Part model, mm, in its own coordinate system. Face numbers are marked on the shaded views. A direction names the side the tool comes from. Round coordinates to 2 decimals unless told otherwise and drop trailing zeros. Write each loop counter-clockwise with the first axis right and the second up, starting at its lowest first coordinate (ties: lowest second). Pieces come first, ordered by that corner, then holes. Notation, with made-up numbers: M 78.25,-7 L 132.25,-7 A31 ccw 132.25,28 Z; hole C -9.75,27.5 d6. An arc over 180 degrees is marked long. Use one line per item in the form item = value. Start each with the question number.
Item 1: Which spindle directions (+Z, -Z, +X, -X, +Y, -Y) get a long thin tool onto all of the face, cutting with end or side? Do the marked faces 5, 6, 7 and 8. Say none if no direction does.
Item 2: Cut at C-C, the plane z = 10.75. Give the cut face in (x, y).
Item 3: Mould opens along Y. For the marked faces 1, 2, 3 and 4 say: +Y half, -Y half, draft (parallel to the pull), parting line (faces both ways), or undercut.
Item 4: Cut at D-D, the plane y = 17. Give the cut face in (x, z).
Item 5: Cut at A-A, the plane z = 4.75. Give the cut face in (x, y).
Item 6: Probe L1, parallel to Y at x = -3, z = 2.5; L2, parallel to X at y = 24.5, z = 3; L3, parallel to Y at x = -18, z = 0.75. List the from-to ranges inside material, lowest first.
Item 7: Flat gauge pins, fed straight in: pin 1 Ø4 at (y, z) = (19, 7.5) entering from +X; pin 2 Ø1.5 at (x, y) = (-5, 18.5) entering from -Z; pin 3 Ø3 at (x, y) = (-20.5, -7) entering from +Z; pin 4 Ø1.2 at (y, z) = (-25.5, 1) entering from +X. Where does each tip first touch, or does it go through?
Item 8: Cut at B-B, the plane x = -4.5. Give the cut face in (y, z), then the cut area to 4 significant figures.
from build123d import *

# Parameters (mm, degrees)
F0_R     = 1.5
F0_W     = 21
F0_H     = 2.5
F0_W_2   = 15.5
F0_W_3   = 6
F0_H_2   = 6
F0_W_4   = 26
F1_DEPTH = 1.5
F2_DEPTH = 9
F3_DEPTH = 2.5
F4_DEPTH = 3
F0_W_5   = 7
F0_H_3   = 12
F0_W_6   = 9
F5_DEPTH = 12.5
F0_W_7   = 11.5
F0_H_4   = 9
F0_W_8   = 2.5
F6_DEPTH = 12.5
F7_W     = 7
F7_H     = 1.5
F8_DEPTH = 45.001


with BuildPart() as f1:
    # F0 (on Top) → F1 (new body)
    with BuildSketch(Plane.XY):
        with BuildLine():
            Line((33, 27), (-33, 27))
            Line((-33, 27), (-33, 18))
            Line((-33, 18), (-24, 18))
            Line((-24, 18), (-24, 6))
            Line((-24, 6), (-33, 6))
            Line((-33, 6), (-33, -14))
            Line((-33, -14), (-21.5, -14))
            Line((-21.5, -14), (-21.5, -23))
            Line((-21.5, -23), (-33, -23))
            Line((-33, -23), (-33, -27))
            Line((-33, -27), (33, -27))
            Line((33, -27), (33, -25))
            Line((33, -25), (33, -21))
            ThreePointArc((33, -21), (31.5, -19.5), (33, -18))
            Line((33, -18), (33, 7.5))
            ThreePointArc((33, 7.5), (31.5, 9), (33, 10.5))
            Line((33, 10.5), (33, 14))
            Line((33, 14), (33, 27))
        make_face()
        with Locations((-19, -24.5)):
            Circle(F0_R, mode=Mode.SUBTRACT)
        with Locations((4, -24.75)):
            Rectangle(F0_W, F0_H, mode=Mode.SUBTRACT)
        with Locations((24.25, -24.75)):
            Rectangle(F0_W_2, F0_H, mode=Mode.SUBTRACT)
        with Locations((-27, 23)):
            Rectangle(F0_W_3, F0_H_2, mode=Mode.SUBTRACT)
        with Locations((-18, 24.5)):
            Circle(F0_R, mode=Mode.SUBTRACT)
        with Locations((-3, 24.75)):
            Rectangle(F0_W_4, F0_H, mode=Mode.SUBTRACT)
        with Locations((21.5, 24.75)):
            Rectangle(F0_W, F0_H, mode=Mode.SUBTRACT)
        with BuildLine():
            Line((36, 11), (33, 14))
            Line((33, 14), (33, 10.5))
            ThreePointArc((33, 10.5), (34.06066, 10.06066), (34.5, 9))
            ThreePointArc((34.5, 9), (34.06066, 7.93934), (33, 7.5))
            Line((33, 7.5), (33, -18))
            ThreePointArc((33, -18), (34.06066, -18.43934), (34.5, -19.5))
            ThreePointArc((34.5, -19.5), (34.06066, -20.56066), (33, -21))
            Line((33, -21), (33, -25))
            Line((33, -25), (36, -22))
            Line((36, -22), (36, 11))
        make_face()
    extrude(amount=F1_DEPTH)

    # F0 (on Top) → F2 (join)
    with BuildSketch(Plane.XY):
        with Locations((-3, 24.75)):
            Rectangle(F0_W_4, F0_H)
        with Locations((21.5, 24.75)):
            Rectangle(F0_W, F0_H)
        with Locations((4, -24.75)):
            Rectangle(F0_W, F0_H)
        with Locations((24.25, -24.75)):
            Rectangle(F0_W_2, F0_H)
    extrude(amount=F2_DEPTH)

    # F0 (on Top) → F3 (join)
    with BuildSketch(Plane.XY):
        with Locations((-27, 23)):
            Rectangle(F0_W_3, F0_H_2)
        with Locations((-27, 23)):
            Circle(F0_R, mode=Mode.SUBTRACT)
    extrude(amount=F3_DEPTH)

    # F0 (on Top) → F4 (join)
    with BuildSketch(Plane.XY):
        with Locations((-27, 23)):
            Circle(F0_R)
    extrude(amount=F4_DEPTH)

    # F0 (on Top) → F5 (join)
    with BuildSketch(Plane.XY):
        with Locations((-36.5, 12)):
            Rectangle(F0_W_5, F0_H_3)
        with Locations((-28.5, 12)):
            Rectangle(F0_W_6, F0_H_3)
    extrude(amount=F5_DEPTH)

    # F0 (on Top) → F6 (join)
    with BuildSketch(Plane.XY):
        with Locations((-27.25, -18.5)):
            Rectangle(F0_W_7, F0_H_4)
        with Locations((-34.25, -18.5)):
            Rectangle(F0_W_8, F0_H_4)
    extrude(amount=F6_DEPTH)

    # F7 (on face) → F8 (cut, through all)
    with BuildSketch(Plane(origin=(0, 18, 0), x_dir=(-1, 0, 0), z_dir=(0, 1, 0))):
        with Locations((36.5, 0.75)):
            Rectangle(F7_W, F7_H)
    extrude(amount=-F8_DEPTH, mode=Mode.SUBTRACT)


solid = f1.part
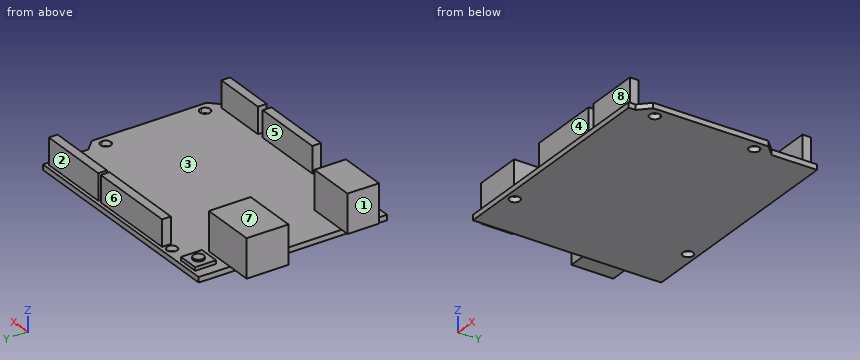
Model answer:
q1.face_5 = +Z, +X, -X
q1.face_6 = +Z, +X, -X, +Y
q1.face_7 = +Z, +X, -X, +Y, -Y
q1.face_8 = +Z, +X, -X, -Y
q2.outline = M -40,6 L -24,6 L -24,18 L -40,18 Z; M -35.5,-23 L -21.5,-23 L -21.5,-14 L -35.5,-14 Z
q3.face_1 = draft
q3.face_2 = +Y half
q3.face_3 = undercut
q3.face_4 = -Y half
q4.outline = M -40,1.5 L -33,1.5 L -33,0 L 33,0 L 33,1.5 L -24,1.5 L -24,12.5 L -40,12.5 Z
q5.outline = M -40,6 L -24,6 L -24,18 L -40,18 Z; M -35.5,-23 L -21.5,-23 L -21.5,-14 L -35.5,-14 Z; M -16,23.5 L 10,23.5 L 10,26 L -16,26 Z; M -6.5,-26 L 14.5,-26 L 14.5,-23.5 L -6.5,-23.5 Z; M 11,23.5 L 32,23.5 L 32,26 L 11,26 Z; M 16.5,-26 L 32,-26 L 32,-23.5 L 16.5,-23.5 Z
q6.L1 = -26 to -23.5, 23.5 to 26
q6.L2 = -16 to 10, 11 to 32
q6.L3 = -27 to -25.62, -23.38 to 23, 26 to 27
q7.pin_1 = -24
q7.pin_2 = 0
q7.pin_3 = 1.5
q7.pin_4 = 33.1
q8.outline = M -27,0 L 27,0 L 27,1.5 L 26,1.5 L 26,9 L 23.5,9 L 23.5,1.5 L -23.5,1.5 L -23.5,9 L -26,9 L -26,1.5 L -27,1.5 Z
q8.area = 118.5 mm²
